```python
from build123d import *

# Parameters (mm, degrees)
SKETCH_1_R      = 2.5
EXTRUDE_2_DEPTH = 100


with BuildPart() as part:
    # 草图1 → 凸台-拉伸2 (new body)
    with BuildSketch(Plane.XY):
        with BuildLine():
            Line((5.5, -8.2), (5.5, -6.560660172))
            Line((5.5, -6.560660172), (2.939339828, -4))
            Line((2.939339828, -4), (-2.939339828, -4))
            Line((-2.939339828, -4), (-5.5, -6.560660172))
            Line((-5.5, -6.560660172), (-5.5, -8.2))
            Line((-5.5, -8.2), (-3.1, -8.2))
            Line((-3.1, -8.2), (-3.1, -10))
            Line((-3.1, -10), (-8.5, -10))
            ThreePointArc((-8.5, -10), (-9.560660172, -9.560660172), (-10, -8.5))
            Line((-10, -8.5), (-10, -3.1))
            Line((-10, -3.1), (-8.2, -3.1))
            Line((-8.2, -3.1), (-8.2, -5.5))
            Line((-8.2, -5.5), (-6.560660172, -5.5))
            Line((-6.560660172, -5.5), (-4, -2.939339828))
            Line((-4, -2.939339828), (-4, 2.939339828))
            Line((-4, 2.939339828), (-6.560660172, 5.5))
            Line((-6.560660172, 5.5), (-8.2, 5.5))
            Line((-8.2, 5.5), (-8.2, 3.1))
            Line((-8.2, 3.1), (-10, 3.1))
            Line((-10, 3.1), (-10, 8.5))
            ThreePointArc((-10, 8.5), (-9.560660172, 9.560660172), (-8.5, 10))
            Line((-8.5, 10), (-3.1, 10))
            Line((-3.1, 10), (-3.1, 8.2))
            Line((-3.1, 8.2), (-5.5, 8.2))
            Line((-5.5, 8.2), (-5.5, 6.560660172))
            Line((-5.5, 6.560660172), (-2.939339828, 4))
            Line((-2.939339828, 4), (2.939339828, 4))
            Line((2.939339828, 4), (5.5, 6.560660172))
            Line((5.5, 6.560660172), (5.5, 8.2))
            Line((5.5, 8.2), (3.1, 8.2))
            Line((3.1, 8.2), (3.1, 10))
            Line((3.1, 10), (8.5, 10))
            ThreePointArc((8.5, 10), (9.560660172, 9.560660172), (10, 8.5))
            Line((10, 8.5), (10, 3.1))
            Line((10, 3.1), (8.2, 3.1))
            Line((8.2, 3.1), (8.2, 5.5))
            Line((8.2, 5.5), (6.560660172, 5.5))
            Line((6.560660172, 5.5), (4, 2.939339828))
            Line((4, 2.939339828), (4, -2.939339828))
            Line((4, -2.939339828), (6.560660172, -5.5))
            Line((6.560660172, -5.5), (8.2, -5.5))
            Line((8.2, -5.5), (8.2, -3.1))
            Line((8.2, -3.1), (10, -3.1))
            Line((10, -3.1), (10, -8.5))
            ThreePointArc((10, -8.5), (9.560660172, -9.560660172), (8.5, -10))
            Line((8.5, -10), (3.1, -10))
            Line((3.1, -10), (3.1, -8.2))
            Line((3.1, -8.2), (5.5, -8.2))
        make_face()
        Circle(SKETCH_1_R, mode=Mode.SUBTRACT)
    extrude(amount=-EXTRUDE_2_DEPTH)


solid = part.part
```
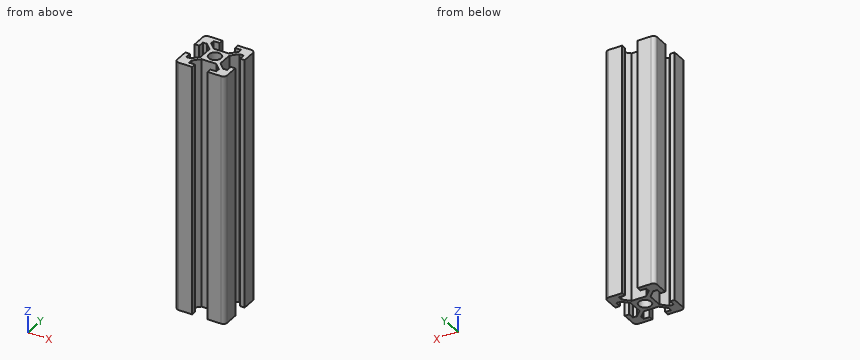
Build history of the part. All positions in model axes, mm. Round coordinates to 2 decimals unless told otherwise and drop trailing zeros. Order: outer loops, then holes, each group sorted by start corner. A loop starts at its lowest first (then second) coordinate and runs counter-clockwise, first axis right, second up. Notation, with made-up numbers: (89, 87) -> (124, 87) arc R13 ccw to (124, 108) -> close; hole circle Ø6 at (60, 89). An arc over 180 degrees is marked (long way). Answer in a Markdown table with one row per item.
1) Pin check, flat tips, straight feed: P1, Ø3, axis at y = 1, z = -34, coming from the -X side; P2, Ø0.9, axis at y = -9.5, z = -32, coming from the +X side; P3, Ø0.5, axis at x = 9.5, z = -52.5, coming from the +Y side. Stop position of each tip, or through.
Values:
| item | result |
|---|---|
| P1 | x = -4 |
| P2 | x = 9.9 |
| P3 | y = 9.8 |
2) Band-saw the part on A-A on y = 0. Give the cut face in (x, z).
Values:
| item | result |
|---|---|
| outline | (-4, -100) -> (-2.5, -100) -> (-2.5, 0) -> (-4, 0) -> close; (2.5, -100) -> (4, -100) -> (4, 0) -> (2.5, 0) -> close |
3) Wall check: L1, parallel to Y at x = 0, z = -68.5; L2, parallel to X at y = 4.75, z = -47.5; L3, parallel to X at y = -5.25, z = -46.5. Give the ranges that are in metal, low to high.
Values:
| item | result |
|---|---|
| L1 | -4 to -2.5, 2.5 to 4 |
| L2 | -10 to -8.2, -5.81 to -3.69, 3.69 to 5.81, 8.2 to 10 |
| L3 | -10 to -8.2, -6.31 to -4.19, 4.19 to 6.31, 8.2 to 10 |
